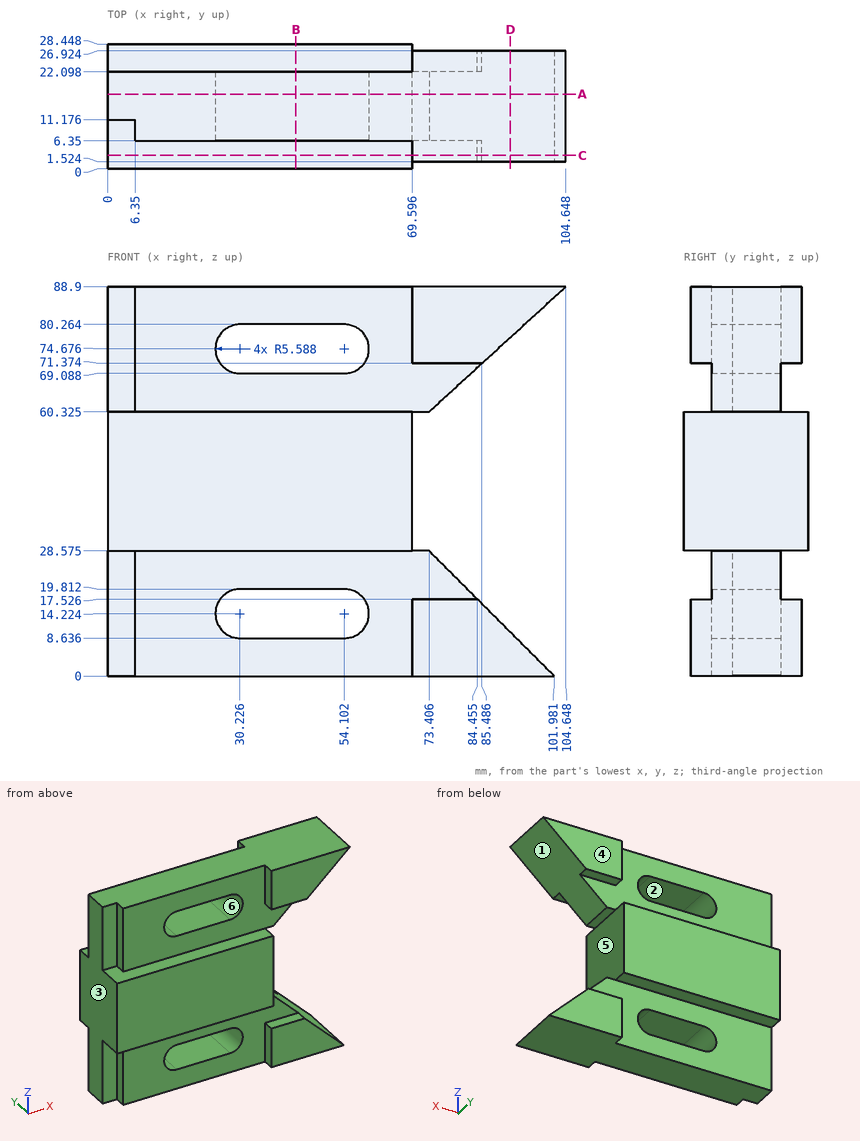
Here's the drawing with two shaded views (mm, measured from the low corner). I have some questions. A direction names the side the tool comes from. Give positions to 0.01 mm unless a question says otherwise; leave off trailing zeros. Loops run counter-clockwise (first coordinate to the right, second up) from the corner with the lowest first, then second, coordinate; pieces in that order, holes last. Notation, with made-up numbers: (67.5, 48.25) - (100.5, 48.25) arc R37 cw to (100.5, 85.25) - close; hole circle Ø9 at (23.5, -31.75). An arc over 180 degrees is marked (long way). Answer in a Markdown table with one row per item. Add a question column.
Q1. If we section it at D-D (x = 92): List the corners of the cut face in (y, z) for me, plus the area to 3 significant figures.
Q2. If we section it at A-A (y = 17): List the corners of the cut face in (x, z) for me (3 decimals).
Q3. If we section it at C-C (y = 3): List the corners of the cut face in (x, z) for me (1 decimal), plus the area to 3 significant figures.
Q4. Please list where these lines run through material, in increasing order: L1, parallel to Z at x = 40, y = 8.5; L2, parallel to Z at x = 28.5, y = 11.5; L3, parallel to Z at x = 12.5, y = 6 (3 decimals). Write a range as from..to.
Q5. Which directions (+Z, -Z, +X, -X, +Y, -Y) give clear straight access to the entire face, cutting with the end or side of a thin tool? Please do the marked faces 1, 2 and 3.
Q6. If we section it at B-B (x = 43): List the corners of the cut face in (y, z) for me (3 decimals).
Q7. We'd pull the mould along X, two halves only. Please class the marked faces 4, 5 and 6: +X half, -X half, draft (parallel to the pull), parting line (faces both ways), or undercut.
Q8. For pin 1 (8.5 mm diameter, centred on x = 50.5, z = 72, fed in from +Y); pin 2 (2.5 mm diameter, centred on y = 8.5, z = 14.5, fed in from -X); pin 3 (2 mm diameter, centred on x = 60, z = 24, fed in from -Y), each with a flat end and sliding along its axis, tell me the tip position at first contact or that it passes through.
The answers:
| question | item | result |
|---|---|---|
| 1 | outline | (1.52, 0) - (26.92, 0) - (26.92, 9.98) - (1.52, 9.98) - close; (1.52, 77.33) - (26.92, 77.33) - (26.92, 88.9) - (1.52, 88.9) - close |
| 1 | area | 547 mm^2 |
| 2 | outline | (0, 0) - (101.981, 0) - (73.406, 28.575) - (69.596, 28.575) - (69.596, 60.325) - (73.406, 60.325) - (104.648, 88.9) - (0, 88.9) - close; hole (30.226, 8.636) - (54.102, 8.636) arc R5.588 ccw to (54.102, 19.812) - (30.226, 19.812) arc R5.588 ccw to start; hole (30.226, 69.088) - (54.102, 69.088) arc R5.588 ccw to (54.102, 80.264) - (30.226, 80.264) arc R5.588 ccw to start |
| 3 | outline | (0, 28.6) - (69.6, 28.6) - (69.6, 60.3) - (0, 60.3) - close; (69.6, 0) - (102, 0) - (84.5, 17.5) - (69.6, 17.5) - close; (69.6, 71.4) - (85.5, 71.4) - (104.6, 88.9) - (69.6, 88.9) - close |
| 3 | area | 3,070 mm^2 |
| 4 | L1 | z = 0..8.64, 19.81..69.09, 80.26..88.9 |
| 4 | L2 | z = 0..8.91, 19.54..69.36, 79.99..88.9 |
| 4 | L3 | z = 28.575..60.325 |
| 5 | face 1 | +X, +Y, -Y |
| 5 | face 2 | +Y, -Y |
| 5 | face 3 | +Z, -Z, -X, +Y, -Y |
| 6 | outline | (0, 28.575) - (6.35, 28.575) - (6.35, 19.812) - (22.098, 19.812) - (22.098, 28.575) - (28.448, 28.575) - (28.448, 60.325) - (22.098, 60.325) - (22.098, 69.088) - (6.35, 69.088) - (6.35, 60.325) - (0, 60.325) - close; (6.35, 0) - (22.098, 0) - (22.098, 8.636) - (6.35, 8.636) - close; (6.35, 80.264) - (22.098, 80.264) - (22.098, 88.9) - (6.35, 88.9) - close |
| 7 | face 4 | draft |
| 7 | face 5 | +X half |
| 7 | face 6 | undercut |
| 8 | pin 1 | stops at y = 22.1 |
| 8 | pin 2 | stops at x = 6.35 |
| 8 | pin 3 | stops at y = 6.35 |
